Verification items for the finished model (mm, model axes). A direction names the side the tool comes from. Round coordinates to 2 decimals unless told otherwise and drop trailing zeros. Order: outer loops, then holes, each group sorted by start corner. A loop starts at its lowest first (then second) coordinate and runs counter-clockwise, first axis right, second up. Notation, with made-up numbers: M 16,-29 L 28,-29 A18 cw 28,-16 Z; hole C 34.5,7 d2. An arc over 180 degrees is marked long. Use one line per item in the form item = value. Start each with the question number.
Item 1: Cross-section at B-B on y = 0.2. Enter the section's corners in (x, z).
Item 2: Thickness scan on probe 1 along X at (y, z) = (1.1, -18); probe 2 along X at (y, z) = (1.1, -42); probe 3 along Z at (x, y) = (81.5, 0.45). Record the ranges inside material, lowest first. Write a range as [from, to].
Item 3: Cross-section at C-C on x = 60. Enter the section's corners in (y, z) (3 decimals), then the cut area to 3 significant figures.
Item 4: Release check for a two-part mould opening along Z. For faces 1 (the cylindrical face through (11.217, 0.579, 26.663)), 2 (the cylindrical face through (10.637, 0.579, -45.133)), 3 (the cylindrical face through (75.865, 0.579, 19.091)), 4 (the flat face through (46, 1.175, -10)) record: +Z half, -Z half, draft (parallel to the pull), parting line (faces both ways), or undercut.
Item 5: Cross-section at A-A on z = -17.5. Enter the section's corners in (x, y) (3 decimals), then the cut area to 3 significant figures.
Item 6: Cross-section at D-D on z = 5.5. Enter the section's corners in (x, y) (3 decimals), then the cut area to 3 significant figures.
Item 7: Tool access check on faces 5 (the cylindrical face through (17.785, 0.579, -38.141)), 6 (the cylindrical face through (83, 0.6, 26.1)). Record the directions out of +Z, -Z, +X, -X, +Y, -Y that give a thin tool (end or side, any length) a straight path to the whole face; none if there is none.
from build123d import *

# Parameters (mm, degrees)
BOSS_EXTRUDE1_DEPTH = 1.175
BOSS_EXTRUDE2_REACH = 127.575
SKETCH4_W           = 19.05
SKETCH4_H           = 1.175


with BuildPart() as part:
    # Sketch1 → Boss-Extrude1 (new body)
    with BuildSketch(Plane(origin=(0, 0, 0), x_dir=(1, 0, 0), z_dir=(0, 1, 0))):
        with BuildLine():
            Line((0, 0), (0, 19.05))
            ThreePointArc((0, 19.05), (10.924917062, 45.425082938), (37.3, 56.35))
            Line((37.3, 56.35), (56.35, 56.35))
            ThreePointArc((56.35, 56.35), (82.725082938, 45.425082938), (93.65, 19.05))
            Line((93.65, 19.05), (93.65, 0))
            ThreePointArc((93.65, 0), (82.725082938, -26.375082938), (56.35, -37.3))
            Line((56.35, -37.3), (37.3, -37.3))
            ThreePointArc((37.3, -37.3), (10.924917062, -26.375082938), (0, 0))
        make_face()
        with BuildLine():
            Line((10, 0), (10, 19.05))
            ThreePointArc((10, 19.05), (17.995984874, 38.354015126), (37.3, 46.35))
            Line((37.3, 46.35), (56.35, 46.35))
            ThreePointArc((56.35, 46.35), (75.654015126, 38.354015126), (83.65, 19.05))
            Line((83.65, 19.05), (83.65, 0))
            ThreePointArc((83.65, 0), (75.654015126, -19.304015126), (56.35, -27.3))
            Line((56.35, -27.3), (37.3, -27.3))
            ThreePointArc((37.3, -27.3), (17.995984874, -19.304015126), (10, 0))
        make_face(mode=Mode.SUBTRACT)
    extrude(amount=BOSS_EXTRUDE1_DEPTH)

    # Boss-Extrude2: up to this face of the body (flat: up to its plane)
    boss_extrude2_end = Plane(part.part.faces().sort_by_distance((46.825, 0.5875, 27.3))[0])
    # Sketch4 → Boss-Extrude2 (add, up to the picked face)
    with BuildSketch(Plane.XY.offset(-46.35), mode=Mode.PRIVATE) as boss_extrude2_sk1:
        with Locations((46.825, 0.5875)):
            Rectangle(SKETCH4_W, SKETCH4_H)
    boss_extrude2_tool1 = split(extrude(boss_extrude2_sk1.sketch, amount=BOSS_EXTRUDE2_REACH, mode=Mode.PRIVATE), bisect_by=boss_extrude2_end, keep=Keep.BOTH, mode=Mode.PRIVATE)
    add(boss_extrude2_tool1.solids().sort_by(Axis((46.825, 0.5875, -46.35), (0, 0, 1)))[0])


solid = part.part
Output values:
q1.outline = M 0,-19.05 A37.3 ccw 37.3,-56.35 L 56.35,-56.35 A37.3 ccw 93.65,-19.05 L 93.65,0 A37.3 ccw 56.35,37.3 L 37.3,37.3 A37.3 ccw 0,0 Z; hole M 10,-19.05 A27.3 ccw 37.3,-46.35 L 37.3,27.3 A27.3 ccw 10,0 Z; hole M 56.35,-46.35 A27.3 ccw 83.65,-19.05 L 83.65,0 A27.3 ccw 56.35,27.3 Z
q2.probe_1 = [0, 10], [37.3, 56.35], [83.65, 93.65]
q2.probe_2 = [7.9, 22.52], [37.3, 56.35], [71.13, 85.75]
q2.probe_3 = [-46.6, -29.67], [10.62, 27.55]
q3.outline = M 0,-56.171 L 1.175,-56.171 L 1.175,-46.105 L 0,-46.105 Z; M 0,27.055 L 1.175,27.055 L 1.175,37.121 L 0,37.121 Z
q3.area = 23.7 mm2
q4.face_1 = +Z half
q4.face_2 = -Z half
q4.face_3 = undercut
q4.face_4 = draft
q5.outline = M 0,0 L 10,0 L 10,1.175 L 0,1.175 Z; M 37.3,0 L 56.35,0 L 56.35,1.175 L 37.3,1.175 Z; M 83.65,0 L 93.65,0 L 93.65,1.175 L 83.65,1.175 Z
q5.area = 45.9 mm2
q6.outline = M 0.408,0 L 10.56,0 L 10.56,1.175 L 0.408,1.175 Z; M 37.3,0 L 56.35,0 L 56.35,1.175 L 37.3,1.175 Z; M 83.09,0 L 93.242,0 L 93.242,1.175 L 83.09,1.175 Z
q6.area = 46.2 mm2
q7.face_5 = +Y, -Y
q7.face_6 = +Z, +X, +Y, -Y
